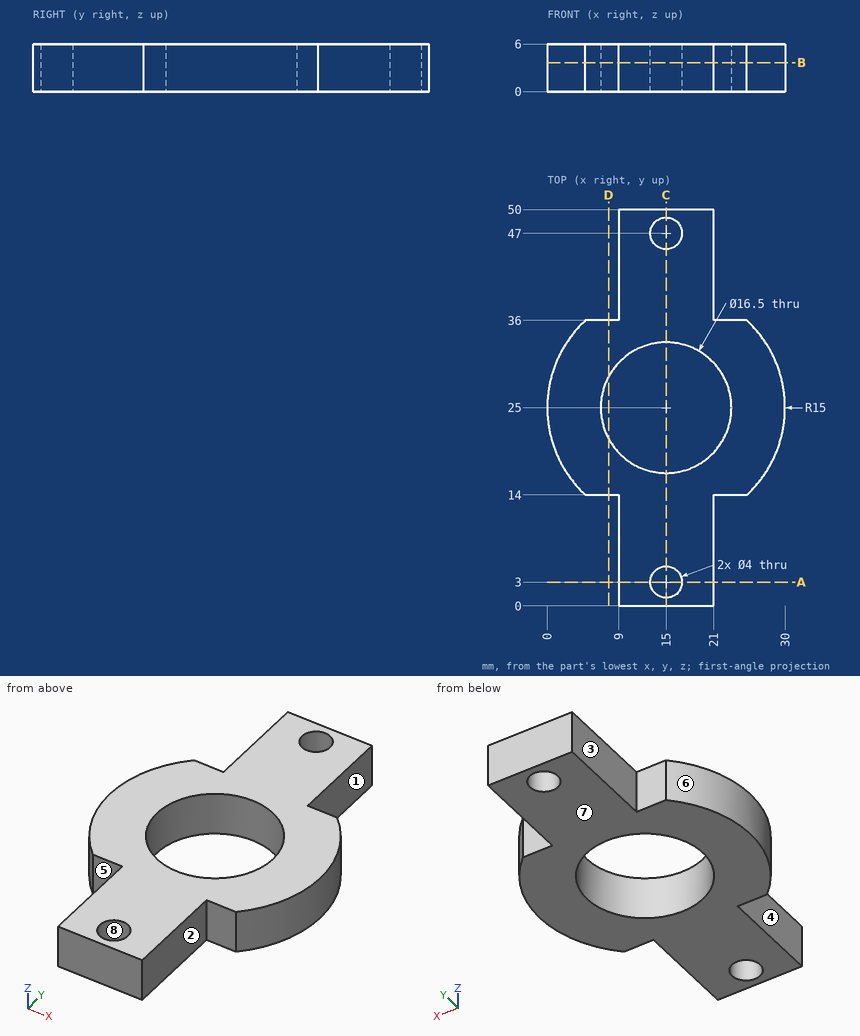
Part print with two shaded views. Sizes in mm from the minimum x, y, z corner. A direction names the side the tool comes from. Give positions to 0.01 mm unless a question says otherwise; leave off trailing zeros. Order: outer loops, then holes, each group sorted by start corner. A loop starts at its lowest first (then second) coordinate and runs counter-clockwise, first axis right, second up. Notation, with made-up numbers: M -19.5,24 L -9.5,24 A15 cw -9.5,46 Z; hole C -28.75,88.5 d3. An arc over 180 degrees is marked long. Put each result on its own line as item: value.
Item 1: Cut at B-B on z = 3.65. Write the cut outline in (x, y), then the cut area to 3 significant figures.
Results are:
outline: M 4.8,14 L 9,14 L 9,0 L 21,0 L 21,14 L 25.2,14 A15 ccw 25.2,36 L 21,36 L 21,50 L 9,50 L 9,36 L 4.8,36 A15 ccw Z; hole C 15,25 d16.5; hole C 15,3 d4; hole C 15,47 d4
area: 692 mm2
Item 2: Cut at D-D on x = 7.75. Write the cut outline in (y, z).
Results are:
outline: M 14,0 L 21.06,0 L 21.06,6 L 14,6 Z; M 28.94,0 L 36,0 L 36,6 L 28.94,6 Z
Item 3: Cut at C-C on x = 15. Write the cut outline in (y, z), then the cut area to 3 significant figures.
Results are:
outline: M 0,0 L 1,0 L 1,6 L 0,6 Z; M 5,0 L 16.75,0 L 16.75,6 L 5,6 Z; M 33.25,0 L 45,0 L 45,6 L 33.25,6 Z; M 49,0 L 50,0 L 50,6 L 49,6 Z
area: 153 mm2
Item 4: Which spindle directions (+Z, -Z, +X, -X, +Y, -Y) get a long thin tool onto all of the face, cutting with end or side? Do the marked faces 1, 2, 3 and 4. Say none if no direction does.
Results are:
face 1: +Z, -Z, +X, +Y
face 2: +Z, -Z, +X, -Y
face 3: +Z, -Z, -X, +Y
face 4: +Z, -Z, -X, -Y
Item 5: Wall check: probe 1 along Y at (x, z) = (15, 4.35); probe 2 along X at (y, z) = (31, 1.2); probe 3 along Y at (x, z) = (11, 5.7). Give the ranges that are in metal, low to high.
Results are:
probe 1: 0 to 1, 5 to 16.75, 33.25 to 45, 49 to 50
probe 2: 1.25 to 9.34, 20.66 to 28.75
probe 3: 0 to 17.78, 32.22 to 50
Item 6: Pull direction Y, two halves, no side cores. Call the marked faces 5, 6, 7 and 8: +Y half, -Y half, draft (parallel to the pull), parting line (faces both ways), or undercut.
Results are:
face 5: -Y half
face 6: parting line
face 7: draft
face 8: undercut
Item 7: Drop flat-ended pins along their axis: pin 1 Ø3 at (x, z) = (7, 2) entering from -Y; pin 2 Ø6.5 at (x, y) = (15, 3) entering from +Z; pin 3 Ø3 at (y, z) = (7, 4.5) entering from +X; pin 4 Ø2 at (y, z) = (42, 2.5) entering from -X. Give the stop position or say it passes through.
Results are:
pin 1: y = 14
pin 2: z = 6
pin 3: x = 21
pin 4: x = 9
Item 8: Cut at A-A on y = 3. Write the cut outline in (x, z), then the cut area to 3 significant figures.
Results are:
outline: M 9,0 L 13,0 L 13,6 L 9,6 Z; M 17,0 L 21,0 L 21,6 L 17,6 Z
area: 48.0 mm2
